Check sheet for the drawn part. Datum: minimum x, y, z corner. Units: mm. Give positions to 0.01 mm unless a question says otherwise; leave off trailing zeros. Write each loop counter-clockwise with the first axis right and the second up, starting at its lowest first coordinate (ties: lowest second). Pieces come first, ordered by that corner, then holes. Notation, with made-up numbers: (-19.5, -12) -> (-3.5, -12) arc R22 ccw to (-3.5, -2) -> close; hole circle Ø3 at (-10.5, 53.5). An arc over 180 degrees is marked (long way). Answer as CSV lines item,"result". Start each with the question number.
1) Sectioned sample at A-A on z = 0.6. Record the cut outline in (x, y), and give its area (3 significant figures).
2) Material ranges on L1, parallel to Y at x = 98, z = 2.85; L2, parallel to X at y = 51, z = 0.25, recorded low to high.
3) Sectioned sample at B-B on x = 22. Record the cut outline in (y, z).
4) Gauge pin test, flat ends, axial feed: pin 1 Ø1 at (x, z) = (108.5, 1) entering from -Y; pin 2 Ø0.9 at (y, z) = (1, 2) entering from -X; pin 3 Ø0.9 at (y, z) = (78, 1.5) entering from +X. Record the tip position at first contact, or that the pin passes through.
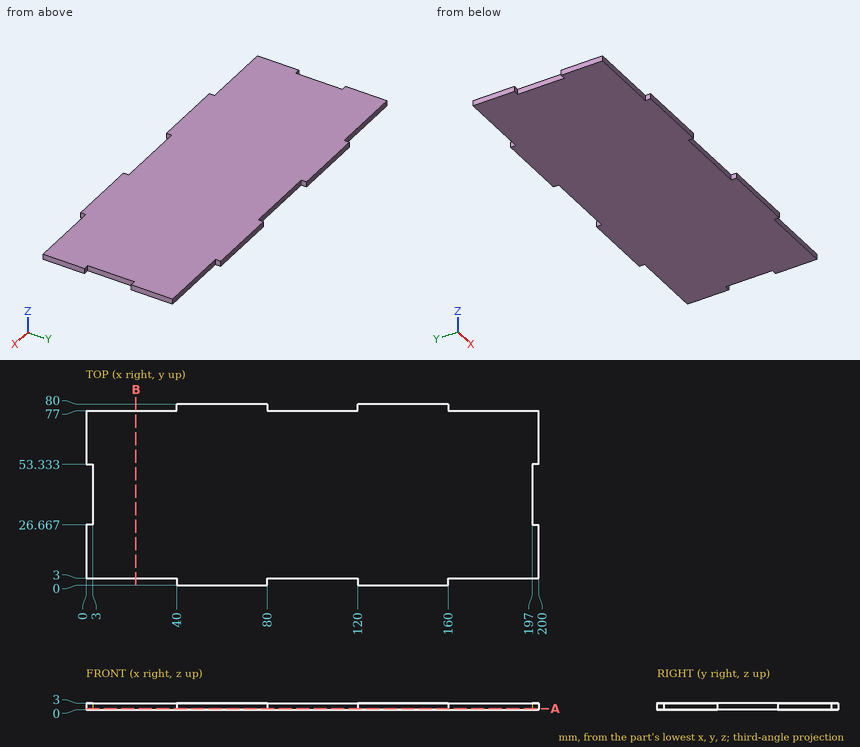
Ans:
1,outline,"(0, 3) -> (40, 3) -> (40, 0) -> (80, 0) -> (80, 3) -> (120, 3) -> (120, 0) -> (160, 0) -> (160, 3) -> (200, 3) -> (200, 26.67) -> (197, 26.67) -> (197, 53.33) -> (200, 53.33) -> (200, 77) -> (160, 77) -> (160, 80) -> (120, 80) -> (120, 77) -> (80, 77) -> (80, 80) -> (40, 80) -> (40, 77) -> (0, 77) -> (0, 53.33) -> (3, 53.33) -> (3, 26.67) -> (0, 26.67) -> close"
1,area,"15,100 mm²"
2,L1,"y = 3 to 77"
2,L2,"x = 3 to 197"
3,outline,"(3, 0) -> (77, 0) -> (77, 3) -> (3, 3) -> close"
4,pin 1,"stops at y = 3"
4,pin 2,"stops at x = 40"
4,pin 3,"stops at x = 160"
